```python
from build123d import *

# Parameters (mm, degrees)
ESBO_O1_R                = 2.79
RESSALTO_EXTRUS_O1_DEPTH = 40.5


with BuildPart() as part:
    # Esboço1 → Ressalto-extrusão1 (new body)
    with BuildSketch(Plane.XZ.offset(34.5)):
        with BuildLine():
            Line((77.062658774, 17.174038106), (78.116878365, 19))
            Line((78.116878365, 19), (77.062658774, 20.825961894))
            ThreePointArc((77.062658774, 20.825961894), (75.013620668, 21.375), (75.562658774, 23.424038106))
            Line((75.562658774, 23.424038106), (74.508439182, 25.25))
            Line((74.508439182, 25.25), (72.4, 25.25))
            ThreePointArc((72.4, 25.25), (70.9, 23.75), (69.4, 25.25))
            Line((69.4, 25.25), (67.291560818, 25.25))
            Line((67.291560818, 25.25), (66.237341226, 23.424038106))
            ThreePointArc((66.237341226, 23.424038106), (66.786379332, 21.375), (64.737341226, 20.825961894))
            Line((64.737341226, 20.825961894), (63.683121635, 19))
            Line((63.683121635, 19), (64.737341226, 17.174038106))
            ThreePointArc((64.737341226, 17.174038106), (66.786379332, 16.625), (66.237341226, 14.575961894))
            Line((66.237341226, 14.575961894), (67.291560818, 12.75))
            Line((67.291560818, 12.75), (69.4, 12.75))
            ThreePointArc((69.4, 12.75), (70.9, 14.25), (72.4, 12.75))
            Line((72.4, 12.75), (74.508439182, 12.75))
            Line((74.508439182, 12.75), (75.562658774, 14.575961894))
            ThreePointArc((75.562658774, 14.575961894), (75.013620668, 16.625), (77.062658774, 17.174038106))
        make_face()
        with Locations(Location((70.9, 19, 0), (0, 0, 90))):
            Circle(ESBO_O1_R, mode=Mode.SUBTRACT)
    extrude(amount=-RESSALTO_EXTRUS_O1_DEPTH)


solid = part.part
```
For this review, take the finished solid that the model builds, in its own axes (mm). Coordinates: 2 decimals unless noted, no trailing zeros. Write each loop counter-clockwise with the first axis right and the second up, starting at its lowest first coordinate (ties: lowest second). Pieces come first, ordered by that corner, then holes.
(1) Add section A-A on x = 70.9. Give the boundary of the cut face in (y, z), then the cut area to 3 significant figures.
(2) For pin 1 Ø1 at (y, z) = (-5, 14) entering from +X; pin 2 Ø1 at (y, z) = (-2, 20.5) entering from -X, all flat-tipped, find the tip position at first contact; note any pin that passes through.
(3) Wall thickness on probe 1 along Z at (x, y) = (70.9, -5); probe 2 along X at (y, z) = (-22, 19); probe 3 along X at (y, z) = (-31, 16): over which ranges is each line inside the solid? List them lowest first.
(4) Add section D-D on z = 22.75. Give the boundary of the cut face in (x, y), then the cut area to 3 significant figures.
(5) Add section B-B on y = -5. Give the boundary of the cut face in (x, z) (3 decimals).
(6) The part is to be moulded in two halves that separate along X. For faces 1 (the face through (66.77, -14.53, 24.35)), 2 (the face through (77.58, -14.53, 18.07)), 3 (the face through (70.87, -14.53, 14.25)), say which applies: +X half, -X half, draft (parallel to the pull), parting line (faces both ways), or undercut.
(7) Add section C-C on z = 20. Give the boundary of the cut face in (x, y), then the cut area to 3 significant figures.
Answer sheet:
1. outline: (-34.5, 14.25) - (6, 14.25) - (6, 16.21) - (-34.5, 16.21) - close; (-34.5, 21.79) - (6, 21.79) - (6, 23.75) - (-34.5, 23.75) - close
1. area: 159 mm2
2. pin 1: stops at x = 75.52
2. pin 2: stops at x = 64.26
3. probe 1: z = 14.25 to 16.21, 21.79 to 23.75
3. probe 2: x = 63.68 to 68.11, 73.69 to 78.12
3. probe 3: x = 66.98 to 74.82
4. outline: (66.85, -34.5) - (74.95, -34.5) - (74.95, 6) - (66.85, 6) - close
4. area: 328 mm2
5. outline: (63.683, 19) - (64.737, 17.174) arc R1.5 cw to (66.237, 14.576) - (67.292, 12.75) - (69.4, 12.75) arc R1.5 cw to (72.4, 12.75) - (74.508, 12.75) - (75.563, 14.576) arc R1.5 cw to (77.063, 17.174) - (78.117, 19) - (77.063, 20.826) arc R1.5 cw to (75.563, 23.424) - (74.508, 25.25) - (72.4, 25.25) arc R1.5 cw to (69.4, 25.25) - (67.292, 25.25) - (66.237, 23.424) arc R1.5 cw to (64.737, 20.826) - close; hole circle Ø5.58 at (70.9, 19)
6. face 1: -X half
6. face 2: +X half
6. face 3: undercut
7. outline: (64.26, -34.5) - (68.3, -34.5) - (68.3, 6) - (64.26, 6) - close; (73.5, -34.5) - (77.54, -34.5) - (77.54, 6) - (73.5, 6) - close
7. area: 327 mm2
